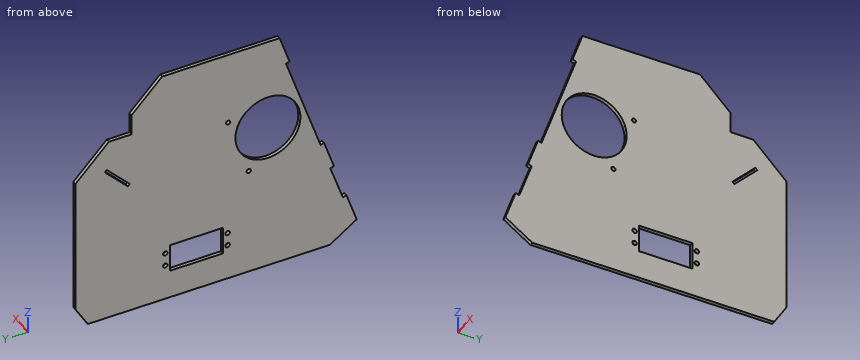
```python
from build123d import *

# Parameters (mm, degrees)
SKETCH1_R           = 1.7
SKETCH1_R_2         = 26
SKETCH1_R_3         = 1.8
SKETCH1_W           = 21.878233713
SKETCH1_H           = 42.578781785
BOSS_EXTRUDE1_DEPTH = 3


with BuildPart() as part:
    # Sketch1 → Boss-Extrude1 (new body)
    with BuildSketch(Plane(origin=(0, 0, 0), x_dir=(0, 0, -1), z_dir=(1, 0, 0))):
        Polygon((-110.882382617, -2.731166398), (-88.223157403, -10.643032479), (-87.23420686, -7.810723029), (-58.937631543, -17.77378609), (-59.926582085, -20.606095541), (-36.324038311, -28.84733785), (-22.003393348, -7.322703446), (-22.003393348, 186.164699152), (-38.083447414, 196.14277913), (-145.230517161, 196.14277913), (-172.036164941, 169.366182911), (-172.036164941, 151.244509979), (-188.398196234, 151.244509979), (-212.871297543, 126.797932251), (-212.871297543, 32.797235558), (-190.212821939, 24.885631216), (-189.235943541, 27.683366592), (-109.931278924, -0.007248606), align=None)
        with Locations((-155.039998164, 73.999598468)):
            Circle(SKETCH1_R, mode=Mode.SUBTRACT)
        with Locations((-107.865704399, 57.52786604)):
            Circle(SKETCH1_R, mode=Mode.SUBTRACT)
        with Locations((-139.694105805, 42.161153499)):
            Circle(SKETCH1_R_2, mode=Mode.SUBTRACT)
        with Locations((-60.718323374, 74.451599653)):
            Circle(SKETCH1_R_3, mode=Mode.SUBTRACT)
        with Locations((-50.368324245, 74.447353909)):
            Circle(SKETCH1_R_3, mode=Mode.SUBTRACT)
        with Locations((-60.697894576, 124.251595463)):
            Circle(SKETCH1_R_3, mode=Mode.SUBTRACT)
        with Locations((-50.347895446, 124.247349719)):
            Circle(SKETCH1_R_3, mode=Mode.SUBTRACT)
        Polygon((-148.535091588, 171.081773838), (-146.971590994, 172.643579934), (-128.596785358, 154.248838352), (-130.160285952, 152.687032257), align=None, mode=Mode.SUBTRACT)
        with Locations((-55.533109411, 99.349474686)):
            Rectangle(SKETCH1_W, SKETCH1_H, mode=Mode.SUBTRACT)
    extrude(amount=BOSS_EXTRUDE1_DEPTH)


solid = part.part
```
Work out the finished part from the listing and answer in its coordinate system (mm). Round coordinates to 2 decimals unless told otherwise and drop trailing zeros. Order: outer loops, then holes, each group sorted by start corner. A loop starts at its lowest first (then second) coordinate and runs counter-clockwise, first axis right, second up.
Q1. A cutting plane is placed at A-A, the plane y = 86.5. Determine the outline of the cut face in (x, z), then the cut area to 3 significant figures.
Solution:
outline: (0, 22) - (3, 22) - (3, 44.59) - (0, 44.59) - close; (0, 66.47) - (3, 66.47) - (3, 212.87) - (0, 212.87) - close
area: 507 mm2
Q2. A cutting plane is placed at D-D, the plane y = 49. Determine the outline of the cut face in (x, z), then the cut area to 3 significant figures.
Solution:
outline: (0, 22) - (3, 22) - (3, 114.61) - (0, 114.61) - close; (0, 164.78) - (3, 164.78) - (3, 212.87) - (0, 212.87) - close
area: 422 mm2
Q3. Given pin 1 Ø1.5 at (x, z) = (2, 179) entering from +Y; pin 2 Ø1.5 at (x, z) = (1.5, 56.5) entering from -Y; pin 3 Ø1.5 at (x, y) = (2, 157) entering from +Z, each flat-ended and moving along its own axis, determine where each tip first touches the part or whether it passes through.
Solution:
pin 1: stops at y = 151.24
pin 2: stops at y = -22.06
pin 3: stops at z = 172.04
Q4. A cutting plane is placed at B-B, the plane z = 137.5. Determine the outline of the cut face in (x, y).
Solution:
outline: (0, 9.62) - (3, 9.62) - (3, 16.25) - (0, 16.25) - close; (0, 68.07) - (3, 68.07) - (3, 160.03) - (0, 160.03) - close; (0, 163.16) - (3, 163.16) - (3, 196.14) - (0, 196.14) - close
Q5. A cutting plane is placed at C-C, the plane x = 1.55. Count the separate pieces of the cut face and the enclosed holes in it, then the cut area to 3 significant figures.
Solution:
separate pieces: 1
enclosed holes: 9
area: 31,300 mm2
Q6. Find the intervals of material crossed by line 1 along Z through (x, y) = (1.9, 57.5); line 2 along Z through (x, y) = (1.3, 153.5); line 3 along Y through (x, z) = (1.95, 52), in increasing order.
Solution:
line 1: z = 22 to 106.17, 109.57 to 118.7, 160.69 to 212.87
line 2: z = 22 to 129.35, 130.97 to 172.04
line 3: y = -23.37 to 73.69, 75.21 to 78.06, 120.64 to 123.53, 124.96 to 196.14
